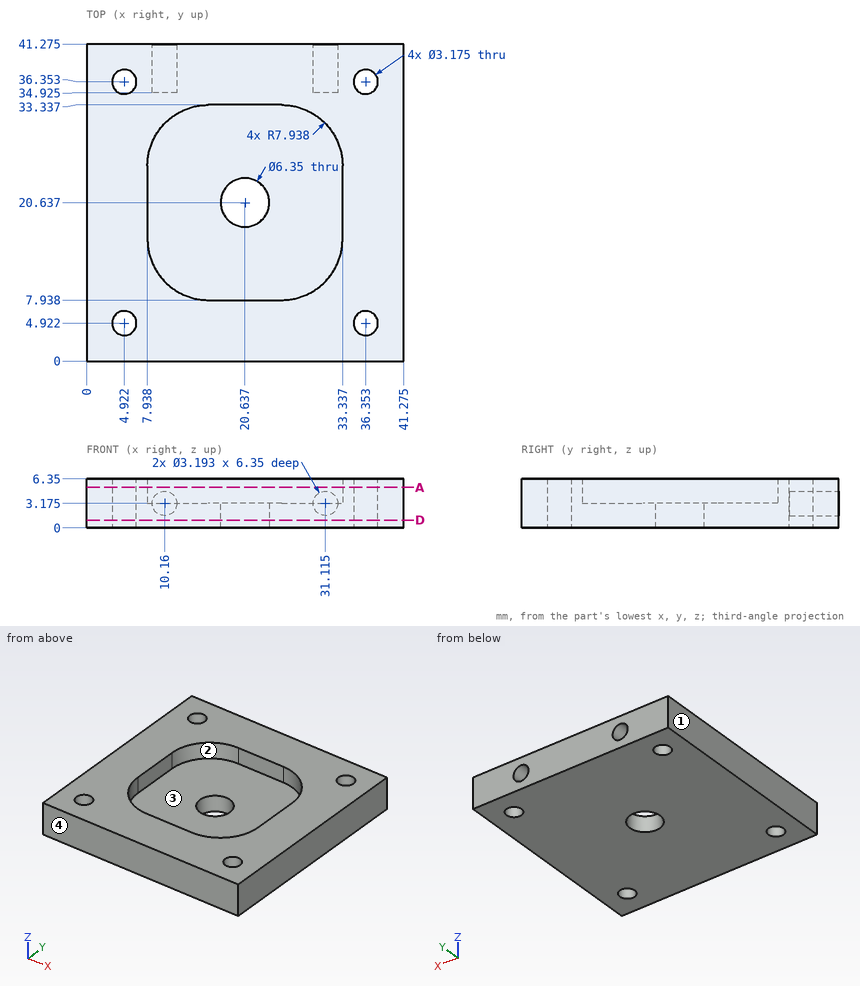
Input: dimensioned drawing with shaded views. Units: mm. Origin: part minimum x, y, z. Round coordinates to 2 decimals unless told otherwise and drop trailing zeros. Loops run counter-clockwise (first coordinate to the right, second up) from the corner with the lowest first, then second, coordinate; pieces in that order, holes last. Notation, with made-up numbers: (89.5, 19.25) -> (128.5, 19.25) arc R31 ccw to (128.5, 45.25) -> close; hole circle Ø11 at (-8, -18.5). An arc over 180 degrees is marked (long way). Use one line per item in the form item = value. Start each with the question number.
1) Section A-A on z = 5.25. Output: boundary loops of the cut face in (x, y) (1 decimal).
2) Line query: L1, parallel to Y at x = 22.5, z = 4 (1 decimal); L2, parallel to X at y = 35.5, z = 5.75 (1 decimal); L3, parallel to X at y = 37, z = 5.25 (1 decimal). Output: solid intervals per line, ascending.
3) Draft query along X for the marked faces 1, 2, 3 and 4. Return one class per face: released by +X, released by -X, zero draft, split by the parting line, or undercut.
4) First-contact query: P1, Ø1.6, axis at x = 31.5, z = 3.5, coming from the +Y side (1 decimal); P2, Ø20.5, axis at x = 17, y = 20.5, coming from the +Z side. Flat tips, straight axial feed; report the tip coordinate or a pass-through.
5) Section D-D on z = 1. Give the number of separate pieces and of enclosed holes in the cut face, then the cut area to 3 significant figures.
Response:
q1.outline = (0, 0) -> (41.3, 0) -> (41.3, 41.3) -> (0, 41.3) -> close; hole circle Ø3.2 at (4.9, 4.9); hole circle Ø3.2 at (4.9, 36.4); hole (7.9, 15.9) arc R7.9 ccw to (15.9, 7.9) -> (25.4, 7.9) arc R7.9 ccw to (33.3, 15.9) -> (33.3, 25.4) arc R7.9 ccw to (25.4, 33.3) -> (15.9, 33.3) arc R7.9 ccw to (7.9, 25.4) -> close; hole circle Ø3.2 at (36.4, 4.9); hole circle Ø3.2 at (36.4, 36.4)
q2.L1 = 0 to 7.9, 33.3 to 41.3
q2.L2 = 0 to 3.6, 6.3 to 35, 37.7 to 41.3
q2.L3 = 0 to 3.5, 6.4 to 34.9, 37.8 to 41.3
q3.face_1 = released by -X
q3.face_2 = undercut
q3.face_3 = undercut
q3.face_4 = zero draft
q4.P1 = 34.9
q4.P2 = 6.35
q5.separate_pieces = 1
q5.enclosed_holes = 5
q5.area = 1,640 mm^2
